Could you check a few things on this model? Use its own coordinates, in mm. A direction names the side the tool comes from. Give positions to 0.01 mm unless a question says otherwise; leave off trailing zeros. Write each loop counter-clockwise with the first axis right and the second up, starting at its lowest first coordinate (ties: lowest second). Pieces come first, ordered by that corner, then holes. Notation, with made-up numbers: (47, 53.25) - (90, 53.25) arc R14 ccw to (90, 63.25) - close; hole circle Ø2 at (-39, 70.5). An arc over 180 degrees is marked (long way). Answer in a Markdown table with one row per item.
from build123d import *

# Parameters (mm, degrees)
SKETCH1_R           = 11
BOSS_EXTRUDE1_DEPTH = 20
SKETCH5_R           = 25
BOSS_EXTRUDE2_DEPTH = 5
CUT_EXTRUDE2_REACH  = 42.62
SKETCH6_R           = 1.5
FILLET2_R           = 5
RIB10_REACH         = 45.301
SKETCH12_WALL_W     = 107.81191309
SKETCH12_WALL_H     = 4
CIRPATTERN1_COUNT   = 4
FILLET3_R           = 1
FILLET4_R           = 0.5
SKETCH13_R          = 3
CUT_EXTRUDE3_DEPTH  = 1
SKETCH14_R          = 1.5
CUT_EXTRUDE4_DEPTH  = 12


with BuildPart() as part:
    # Sketch1 → Boss-Extrude1 (new body)
    with BuildSketch(Plane.XY):
        Circle(SKETCH1_R)
    extrude(amount=BOSS_EXTRUDE1_DEPTH)

    # Sketch5 → Boss-Extrude2 (add)
    with BuildSketch(Plane.XY.offset(20)):
        Circle(SKETCH5_R)
    extrude(amount=BOSS_EXTRUDE2_DEPTH)

    # Sketch6 → Cut-Extrude2 (cut, up to next)
    with BuildSketch(Plane(origin=(0, 0, 20), x_dir=(-1, 0, 0), z_dir=(0, 0, -1)), mode=Mode.PRIVATE) as cut_extrude2_sk1:
        with Locations((0, 20)):
            Circle(SKETCH6_R)
    cut_extrude2_tool1 = extrude(cut_extrude2_sk1.sketch, amount=-CUT_EXTRUDE2_REACH, mode=Mode.PRIVATE) & part.part
    # Sketch6 → Cut-Extrude2 (cut, up to next)
    with BuildSketch(Plane(origin=(0, 0, 20), x_dir=(-1, 0, 0), z_dir=(0, 0, -1)), mode=Mode.PRIVATE) as cut_extrude2_sk2:
        with Locations((0, -20)):
            Circle(SKETCH6_R)
    cut_extrude2_tool2 = extrude(cut_extrude2_sk2.sketch, amount=-CUT_EXTRUDE2_REACH, mode=Mode.PRIVATE) & part.part
    # Sketch6 → Cut-Extrude2 (cut, up to next)
    with BuildSketch(Plane(origin=(0, 0, 20), x_dir=(-1, 0, 0), z_dir=(0, 0, -1)), mode=Mode.PRIVATE) as cut_extrude2_sk3:
        with Locations((-20, 0)):
            Circle(SKETCH6_R)
    cut_extrude2_tool3 = extrude(cut_extrude2_sk3.sketch, amount=-CUT_EXTRUDE2_REACH, mode=Mode.PRIVATE) & part.part
    # Sketch6 → Cut-Extrude2 (cut, up to next)
    with BuildSketch(Plane(origin=(0, 0, 20), x_dir=(-1, 0, 0), z_dir=(0, 0, -1)), mode=Mode.PRIVATE) as cut_extrude2_sk4:
        with Locations((20, 0)):
            Circle(SKETCH6_R)
    cut_extrude2_tool4 = extrude(cut_extrude2_sk4.sketch, amount=-CUT_EXTRUDE2_REACH, mode=Mode.PRIVATE) & part.part
    add(cut_extrude2_tool1.solids().sort_by_distance((0, 20, 20))[0], mode=Mode.SUBTRACT)
    add(cut_extrude2_tool2.solids().sort_by_distance((0, -20, 20))[0], mode=Mode.SUBTRACT)
    add(cut_extrude2_tool3.solids().sort_by_distance((20, 0, 20))[0], mode=Mode.SUBTRACT)
    add(cut_extrude2_tool4.solids().sort_by_distance((-20, 0, 20))[0], mode=Mode.SUBTRACT)

    # Fillet2
    fillet2_edges = [part.edges().sort_by_distance(p)[0] for p in [
        (-11, 0, 20),
    ]]
    fillet(fillet2_edges, radius=FILLET2_R)

    # Sketch12 wall → Rib10 (add, up to next)
    with BuildSketch(Plane(origin=(12.02081528, 12.02081528, 12.5), x_dir=(0.441726104292, 0.441726104292, 0.780868809452), z_dir=(0.55215763038, 0.55215763038, -0.624695047544)), mode=Mode.PRIVATE) as rib10_sk1:
        Rectangle(SKETCH12_WALL_W, SKETCH12_WALL_H)
    rib10_tool1 = extrude(rib10_sk1.sketch, amount=-RIB10_REACH, mode=Mode.PRIVATE) - part.part
    rib10 = rib10_tool1.solids().sort_by_distance((12.02081528, 12.02081528, 12.5))[0]
    add(rib10)

    # CirPattern1: Rib10 ×4 about axis
    cirpattern1_axis = Axis((0, 0, 0), (0, 0, 1))
    for i in range(1, CIRPATTERN1_COUNT):
        add(rib10.rotate(cirpattern1_axis, i * 360 / CIRPATTERN1_COUNT))

    # Fillet3
    fillet3_edges = [part.edges().sort_by_distance(p)[0] for p in [
        (-25, 0, 20),
    ]]
    fillet(fillet3_edges, radius=FILLET3_R)

    # Fillet4
    fillet4_edges = [part.edges().sort_by_distance(p)[0] for p in [
        (10.541779056, -13.370206181, 12.385408642),
        (13.370206181, -10.541779056, 12.385408642),
        (-10.541779056, -13.370206181, 12.385408642),
        (-13.370206181, -10.541779056, 12.385408642),
        (13.370206181, 10.541779056, 12.385408642),
        (10.541779056, 13.370206181, 12.385408642),
        (-13.370206181, 10.541779056, 12.385408642),
        (-10.541779056, 13.370206181, 12.385408642),
    ]]
    fillet(fillet4_edges, radius=FILLET4_R)

    # Sketch13 → Cut-Extrude3 (cut)
    with BuildSketch(Plane(origin=(0, 0, 20), x_dir=(-1, 0, 0), z_dir=(0, 0, -1))):
        with Locations((-20, 0)):
            Circle(SKETCH13_R)
        with Locations((0, 20)):
            Circle(SKETCH13_R)
        with Locations((20, 0)):
            Circle(SKETCH13_R)
        with Locations((0, -20)):
            Circle(SKETCH13_R)
    extrude(amount=-CUT_EXTRUDE3_DEPTH, mode=Mode.SUBTRACT)

    # Sketch14 → Cut-Extrude4 (cut)
    with BuildSketch(Plane(origin=(0, 0, 0), x_dir=(-1, 0, 0), z_dir=(0, 0, -1))):
        with Locations((-5.656854249, 5.656854249)):
            Circle(SKETCH14_R)
        with Locations((5.656854249, -5.656854249)):
            Circle(SKETCH14_R)
        with Locations((5.656854249, 5.656854249)):
            Circle(SKETCH14_R)
        with Locations(Location((-5.656854249, -5.656854249, 0), (0, 0, 180))):
            Circle(SKETCH14_R)
    extrude(amount=-CUT_EXTRUDE4_DEPTH, mode=Mode.SUBTRACT)


solid = part.part
1) If I drill on line 1 (Y direction, x = 7, z = 8.5); line 2 (X direction, y = -0.5, z = 24) (3 decimals); line 3 (Y direction, x = -20, z = 20.4), over which ranges is the centre line in solid material (lowest first)?
Check values:
| item | result |
|---|---|
| line 1 | y = -9.83 to -6.32, -4.99 to 4.99, 6.32 to 9.83 |
| line 2 | x = -24.995 to -21.414, -18.586 to 18.586, 21.414 to 24.995 |
| line 3 | y = -14.66 to -3, 3 to 14.66 |
2) On a 3-axis mill with a long thin cutter (end or side, diameter ignored), from which of +Z, -Z, +X, -X, +Y, -Y can I reach the whole of each face in a straight line? I mean faces 4 (the face through (11.62, 8.79, 14.35)), 5 (the face through (11.91, -11.94, 12.33)), 6 (the face through (0.65, 17.07, 20.49)). Say none if no direction works.
Check values:
| item | result |
|---|---|
| face 4 | -Z, +X |
| face 5 | -Z, +X, -Y |
| face 6 | -Z |
3) We'd pull the mould along X, two halves only. Please class faces 1 (the face through (-13.272, -10.646, 12.631)), 2 (the face through (11.62, -8.79, 14.35)), 3 (the face through (0.195, -18.513, 22.972)): +X half, -X half, draft (parallel to the pull), parting line (faces both ways), or undercut.
Check values:
| item | result |
|---|---|
| face 1 | -X half |
| face 2 | +X half |
| face 3 | undercut |
4) Imagine slicing it at A-A (x = 0). List the corners of the cut face in (y, z) for me.
Check values:
| item | result |
|---|---|
| outline | (-25, 21) arc R1 ccw to (-24, 20) - (-23, 20) - (-23, 21) - (-21.5, 21) - (-21.5, 25) - (-25, 25) - close; (-18.5, 21) - (-17, 21) - (-17, 20) - (-16, 20) arc R5 cw to (-11, 15) - (-11, 0) - (11, 0) - (11, 15) arc R5 cw to (16, 20) - (17, 20) - (17, 21) - (18.5, 21) - (18.5, 25) - (-18.5, 25) - close; (21.5, 21) - (23, 21) - (23, 20) - (24, 20) arc R1 ccw to (25, 21) - (25, 25) - (21.5, 25) - close |
5) Will these pins go through, and if not, where does the flat tip stop? P1, Ø1.8, axis at x = 0, y = -20, coming from the +Z side; P2, Ø6, axis at y = -5.5, z = 12, coming from the +X side; P3, Ø3.5, axis at x = 20, y = 0, coming from the -Z side; P4, Ø2.5, axis at x = -5.66, y = -5.66, coming from the -Z side.
Check values:
| item | result |
|---|---|
| P1 | passes through |
| P2 | stops at x = 11.33 |
| P3 | stops at z = 21 |
| P4 | stops at z = 12 |
